Here's how the part is built. I have some questions about the finished solid (model axes, mm). A direction names the side the tool comes from. Give positions to 0.01 mm unless a question says otherwise; leave off trailing zeros. Order: outer loops, then holes, each group sorted by start corner. A loop starts at its lowest first (then second) coordinate and runs counter-clockwise, first axis right, second up.
from build123d import *

# Parameters (mm, degrees)
F0_W      = 101.6
F0_H      = 50.8
F1_DEPTH  = 50.8
F3_DEPTH  = 59.69
F4_DEPTH  = 12.7
F6_DEPTH  = 12.7
F7_R      = 6.35
F8_DEPTH  = 67.818
F9_R      = 6.35
F10_DEPTH = 76.2


with BuildPart() as f1:
    # F0 (on Top) → F1 (new body)
    with BuildSketch(Plane.XY):
        with Locations((-12.215394, -1.520658)):
            Rectangle(F0_W, F0_H)
    extrude(amount=F1_DEPTH)

    # F2 (on face) → F3 (cut)
    with BuildSketch(Plane.XZ.offset(26.920658)):
        with BuildLine():
            Line((-0.523097, 50.8), (-23.907691, 50.8))
            ThreePointArc((-23.907691, 50.8), (-12.215394, 39.107703), (-0.523097, 50.8))
        make_face()
    extrude(amount=-F3_DEPTH, mode=Mode.SUBTRACT)

    # F2 (on face) → F4 (join)
    with BuildSketch(Plane.XZ.offset(26.920658)):
        with BuildLine():
            Line((-23.907691, 50.8), (-29.430878, 50.8))
            ThreePointArc((-29.430878, 50.8), (-12.215394, 33.584516), (5.00009, 50.8))
            Line((5.00009, 50.8), (-0.523097, 50.8))
            ThreePointArc((-0.523097, 50.8), (-12.215394, 39.107703), (-23.907691, 50.8))
        make_face()
    extrude(amount=F4_DEPTH)

    # F5 (on face) → F6 (join)
    with BuildSketch(Plane(origin=(0, 23.879342, 0), x_dir=(-1, 0, 0), z_dir=(0, 1, 0))):
        with BuildLine():
            Line((0.523097, 50.8), (-4.988703, 50.8))
            ThreePointArc((-4.988703, 50.8), (12.215394, 33.595903), (29.419491, 50.8))
            Line((29.419491, 50.8), (23.907691, 50.8))
            ThreePointArc((23.907691, 50.8), (12.215394, 39.107703), (0.523097, 50.8))
        make_face()
    extrude(amount=F6_DEPTH)

    # F7 (on face) → F8 (cut)
    with BuildSketch(Plane.XY.offset(50.8)):
        with Locations((-46.217443, -1.520658)):
            Circle(F7_R)
    extrude(amount=-F8_DEPTH, mode=Mode.SUBTRACT)

    # F9 (on face) → F10 (cut)
    with BuildSketch(Plane.XY.offset(50.8)):
        with Locations((21.786655, -1.520658)):
            Circle(F9_R)
    extrude(amount=-F10_DEPTH, mode=Mode.SUBTRACT)


solid = f1.part
Q1. For faces 1 (the face through (-11.8, 30.1, 33.6)), 2 (the face through (-12.59, -33.18, 33.59)), 3 (the face through (-44, 6, 50.8)), which set-ups out of +Z, -Z, +X, -X, +Y, -Y let a thin tool reach every point of the face, with its end or its side?
Filled sheet:
face 1: -Z, +Y
face 2: -Z, -Y
face 3: +Z, +X, -X, +Y, -Y
Q2. I'm going to push flat-ended pins straight in: P1, Ø1, axis at x = 24, z = 38, coming from the -Y side; P2, Ø10, axis at x = 21.79, y = -1.52, coming from the +Z side; P3, Ø1, axis at x = 20.5, z = 31.5, coming from the +Y side. Where does each tip first touch, or does it pass through?
Filled sheet:
P1: stops at y = -26.92
P2: passes through
P3: stops at y = 23.88
Q3. If we section it at C-C on y = -14: List the corners of the cut face in (x, z) for me.
Filled sheet:
outline: (-63.02, 0) - (38.58, 0) - (38.58, 50.8) - (-0.52, 50.8) arc R11.69 cw to (-23.91, 50.8) - (-63.02, 50.8) - close
Q4. If we section it at B-B on z = 43: List the corners of the cut face in (x, y) for me.
Filled sheet:
outline: (-63.02, -26.92) - (-27.56, -26.92) - (-27.56, -39.62) - (-20.93, -39.62) - (-20.93, 36.58) - (-27.55, 36.58) - (-27.55, 23.88) - (-63.02, 23.88) - close; (-3.51, -39.62) - (3.13, -39.62) - (3.13, -26.92) - (38.58, -26.92) - (38.58, 23.88) - (3.12, 23.88) - (3.12, 36.58) - (-3.51, 36.58) - close; hole circle Ø12.7 at (-46.22, -1.52); hole circle Ø12.7 at (21.79, -1.52)
Q5. If we section it at D-D on x = -17: List the corners of the cut face in (y, z) for me, plus the area to 3 significant figures.
Filled sheet:
outline: (-39.62, 34.26) - (-26.92, 34.26) - (-26.92, 0) - (23.88, 0) - (23.88, 34.27) - (36.58, 34.27) - (36.58, 40.13) - (-39.62, 40.13) - close
area: 2,190 mm2
Q6. I need wall thicknesses on L1, parallel to Y at x = -46, z = 45; L2, parallel to X at y = 0, z = 12; L3, parallel to X at y = -6, z = 10. Which ranges of each line are inside material? Lowest first, please.
Filled sheet:
L1: y = -26.92 to -7.87, 4.83 to 23.88
L2: x = -63.02 to -52.38, -40.05 to 15.62, 27.95 to 38.58
L3: x = -63.02 to -50.72, -41.72 to 17.29, 26.29 to 38.58
Q7. Thinking about a two-plate mould opening in Y: for faces 4 (the face through (38.585, -2, 25)), 5 (the face through (-52.56, -1.24, 25.76)), 6 (the face through (16.748, -5.385, 25.756)), 7 (the face through (-13, -26.921, 25)), which applies, released by +Y, released by -Y, zero draft, split by the parting line, or undercut?
Filled sheet:
face 4: zero draft
face 5: undercut
face 6: undercut
face 7: released by -Y
Q8. If we section it at A-A on x = -50.5: List the corners of the cut face in (y, z) for me, plus the area to 3 significant figures.
Filled sheet:
outline: (-26.92, 0) - (-6.21, 0) - (-6.21, 50.8) - (-26.92, 50.8) - close; (3.17, 0) - (23.88, 0) - (23.88, 50.8) - (3.17, 50.8) - close
area: 2,100 mm2
